The model under review builds one solid part; all positions refer to its coordinate system, in mm. Face numbers are marked on the shaded views. Round coordinates to 2 decimals unless told otherwise and drop trailing zeros. Order: outer loops, then holes, each group sorted by start corner. A loop starts at its lowest first (then second) coordinate and runs counter-clockwise, first axis right, second up. Notation, with made-up numbers: M 27.5,85 L 63.5,85 A24 ccw 63.5,123 Z; hole C -3,-24.75 d8. An arc over 180 degrees is marked long. Answer as a JSON object with one key per item and string values. Group by question number.
1. Add section A-A on z = -7.5. State the section outline as (x, y) points.
2. To check wall thickness, follow probe 1 along X at (y, z) = (-150.5, -8); probe 2 along Y at (x, z) = (-110, -2); probe 3 along Z at (x, y) = (-141, 36). State the ranges of each line that lie inside material, in increasing order. Write a range as [from, to].
3. Add section C-C on x = 12. State the section outline as (y, z) points.
4. Clearance check with flat-ended pins moving along their axes: P1, Ø5, axis at y = -22, z = -3.5, coming from the -X side; P2, Ø1, axis at y = -70.5, z = -5.5, coming from the +X side; P3, Ø1, axis at x = -81.5, z = -8.5, coming from the +Y side. State where each tip first meets the part, or that it passes through.
5. Mouldability with a two-part tool opening along Y and no side actions: class the marked faces 1 and 2 as released by +Y, released by -Y, zero draft, split by the parting line, or undercut.
6. Add section B-B on y = 100. State the section outline as (x, z) points, and give its area (3 significant figures).
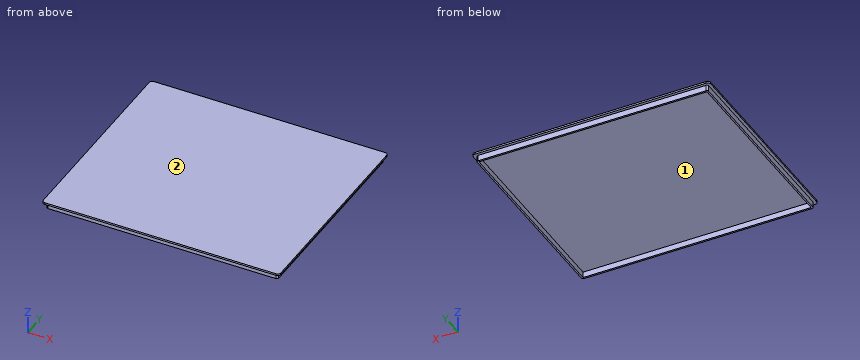
```python
from build123d import *

# Parameters (mm, degrees)
F0_W     = 394
F0_H     = 343
F0_W_2   = 388
F0_H_2   = 337
F1_DEPTH = 10
F2_W     = 404
F2_H     = 353
F3_DEPTH = 3
F4_R     = 5
F5_R     = 3


with BuildPart() as f1:
    # F0 (on Top) → F1 (new body)
    with BuildSketch(Plane.XY):
        Rectangle(F0_W, F0_H)
        Rectangle(F0_W_2, F0_H_2, mode=Mode.SUBTRACT)
    extrude(amount=-F1_DEPTH)

    # F2 (on face) → F3 (join)
    with BuildSketch(Plane.XY):
        Rectangle(F2_W, F2_H)
    extrude(amount=F3_DEPTH)

    # F4
    f4_edges = [f1.edges().sort_by_distance(p)[0] for p in [
        (-202, -176.5, 1.5),
        (202, -176.5, 1.5),
        (202, 176.5, 1.5),
        (-202, 176.5, 1.5),
    ]]
    fillet(f4_edges, radius=F4_R)

    # F5
    f5_edges = [f1.edges().sort_by_distance(p)[0] for p in [
        (197, 171.5, -5),
        (-197, 171.5, -5),
        (-197, -171.5, -5),
        (197, -171.5, -5),
    ]]
    fillet(f5_edges, radius=F5_R)


solid = f1.part
```
Recorded:
{
 "1": {"outline": "M -197,-168.5 A3 ccw -194,-171.5 L 194,-171.5 A3 ccw 197,-168.5 L 197,168.5 A3 ccw 194,171.5 L -194,171.5 A3 ccw -197,168.5 Z; hole M -194,-168.5 L 194,-168.5 L 194,168.5 L -194,168.5 Z"},
 "2": {"probe 1": "x = [-197, -194], [194, 197]", "probe 2": "y = [-171.5, -168.5], [168.5, 171.5]", "probe 3": "z = [0, 3]"},
 "3": {"outline": "M -176.5,0 L -171.5,0 L -171.5,-10 L -168.5,-10 L -168.5,0 L 168.5,0 L 168.5,-10 L 171.5,-10 L 171.5,0 L 176.5,0 L 176.5,3 L -176.5,3 Z"},
 "4": {"P1": "stops at x = -197", "P2": "stops at x = 197", "P3": "stops at y = 171.5"},
 "5": {"face 1": "undercut", "face 2": "zero draft"},
 "6": {"outline": "M -202,0 L -197,0 L -197,-10 L -194,-10 L -194,0 L 194,0 L 194,-10 L 197,-10 L 197,0 L 202,0 L 202,3 L -202,3 Z", "area": "1,270 mm²"}
}
